Verification items for the finished model (mm, model axes). Face numbers are marked on the shaded views. A direction names the side the tool comes from. Round coordinates to 2 decimals unless told otherwise and drop trailing zeros. Order: outer loops, then holes, each group sorted by start corner. A loop starts at its lowest first (then second) coordinate and runs counter-clockwise, first axis right, second up. Notation, with made-up numbers: M -20,52.5 L 32,52.5 A21 ccw 32,80.5 Z; hole C 23.25,8.25 d9. An arc over 180 degrees is marked long. One line per item, written item: value. Start each with the question number.
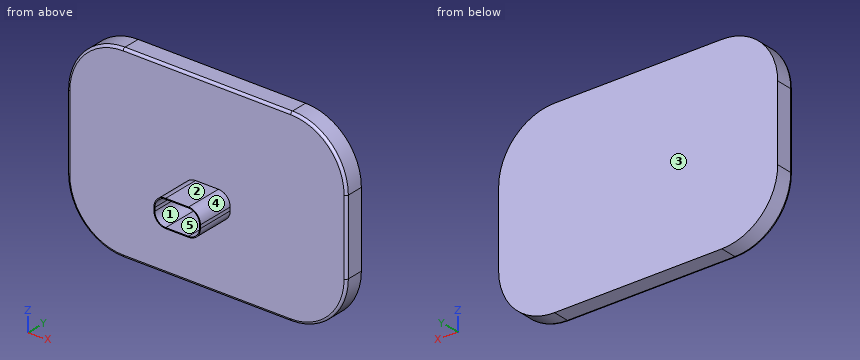
from build123d import *

# Parameters (mm, degrees)
F1_DEPTH = 20
F3_DEPTH = 40
F4_T     = -1
F5_R     = 2.54


with BuildPart() as f1:
    # F0 (on Front) → F1 (new body)
    with BuildSketch(Plane.XZ):
        with BuildLine():
            ThreePointArc((0, 60), (17.5735931288, 17.5735931288), (60, 0))
            Line((60, 0), (240, 0))
            ThreePointArc((240, 0), (282.4264068712, 17.5735931288), (300, 60))
            Line((300, 60), (300, 140))
            ThreePointArc((300, 140), (282.4264068712, 182.4264068712), (240, 200))
            Line((240, 200), (60, 200))
            ThreePointArc((60, 200), (17.5735931288, 182.4264068712), (0, 140))
            Line((0, 140), (0, 60))
        make_face()
    extrude(amount=F1_DEPTH)

    # F2 (on face) → F3 (join)
    with BuildSketch(Plane.XZ.offset(20)):
        with BuildLine():
            Line((175, 83.7), (175, 85.5))
            Line((175, 85.5), (175, 87.3))
            ThreePointArc((175, 87.3), (171.2802561211, 96.2802561211), (162.3, 100))
            Line((162.3, 100), (150, 100))
            Line((150, 100), (137.7, 100))
            ThreePointArc((137.7, 100), (128.7197438789, 96.2802561211), (125, 87.3))
            Line((125, 87.3), (125, 85.5))
            Line((125, 85.5), (125, 83.7))
            ThreePointArc((125, 83.7), (128.7197438789, 74.7197438789), (137.7, 71))
            Line((137.7, 71), (162.3, 71))
            ThreePointArc((162.3, 71), (171.2802561211, 74.7197438789), (175, 83.7))
        make_face()
    extrude(amount=F3_DEPTH)

    # F4
    f4_openings = [f1.faces().sort_by_distance(p)[0] for p in [
        (150, -60, 85.5),
    ]]
    offset(amount=F4_T, openings=f4_openings, kind=Kind.INTERSECTION)

    # F5
    f5_edges = [f1.edges().sort_by_distance(p)[0] for p in [
        (300, -20, 100),
        (150, -20, 200),
        (0, -20, 100),
        (150, -20, 0),
    ]]
    fillet(f5_edges, radius=F5_R)


solid = f1.part
1. Section check D-D (y = -36.5). Record the cut outline in (x, z).
2. Section check C-C (x = 159). Record the cut outline in (y, z), and give its area (3 significant figures).
3. Section check B-B (x = 196). Record the cut outline in (y, z), and give its area (3 significant figures).
4. Tool access check on the marked faces 4 and 5. Record the directions out of +Z, -Z, +X, -X, +Y, -Y that give a thin tool (end or side, any length) a straight path to the whole face; none if there is none.
5. Depth check by flat-ended pin: pin 1 (4 mm diameter, centred on y = -49, z = 87, fed in from +X); pin 2 (12 mm diameter, centred on x = 36, y = -15.5, fed in from +Z); pin 3 (5 mm diameter, centred on x = 115.5, z = 33.5, fed in from -Y); pin 4 (4 mm diameter, centred on y = -52, z = 67.5, fed in from +X). Enter the tip coordinate at first touch or a pass-through.
6. Scan lines: line 1 along Y through (x, z) = (135, 64.5); line 2 along Z through (x, y) = (169.5, -16); line 3 along X through (y, z) = (-5.5, 92.5). Record each from-to range of solid material in increasing order.
7. Section check A-A (y = -6). Record the cut outline in (x, z), and give its area (3 significant figures).
8. Draft check along Z on the marked faces 1, 2 and 3. Enter one of: released by +Z, released by -Z, zero draft, split by the parting line, or undercut.
Geometry check:
1. outline: M 125,83.7 A12.7 ccw 137.7,71 L 162.3,71 A12.7 ccw 175,83.7 L 175,87.3 A12.7 ccw 162.3,100 L 137.7,100 A12.7 ccw 125,87.3 Z; hole M 126,83.7 A11.7 ccw 137.7,72 L 162.3,72 A11.7 ccw 174,83.7 L 174,87.3 A11.7 ccw 162.3,99 L 137.7,99 A11.7 ccw 126,87.3 Z
2. outline: M -60,71 L -20,71 L -20,2.54 A2.54 ccw -17.46,0 L 0,0 L 0,200 L -17.46,200 A2.54 ccw -20,197.46 L -20,100 L -60,100 L -60,99 L -19,99 L -19,199 L -1,199 L -1,1 L -19,1 L -19,72 L -60,72 Z
2. area: 486 mm²
3. outline: M -20,2.54 A2.54 ccw -17.46,0 L 0,0 L 0,200 L -17.46,200 A2.54 ccw -20,197.46 Z; hole M -19,1 L -1,1 L -1,199 L -19,199 Z
3. area: 433 mm²
4. face 4: +Z, +X, -Y
4. face 5: -Y
5. pin 1: stops at x = 175
5. pin 2: stops at z = 197.24
5. pin 3: stops at y = -20
5. pin 4: passes through
6. line 1: y = -20 to -19, -1 to 0
6. line 2: z = 0 to 1, 199 to 200
6. line 3: x = 0 to 1, 299 to 300
7. outline: M 0,60 A60 ccw 60,0 L 240,0 A60 ccw 300,60 L 300,140 A60 ccw 240,200 L 60,200 A60 ccw 0,140 Z; hole M 1,60 A59 ccw 60,1 L 240,1 A59 ccw 299,60 L 299,140 A59 ccw 240,199 L 60,199 A59 ccw 1,140 Z
7. area: 894 mm²
8. face 1: undercut
8. face 2: released by +Z
8. face 3: zero draft
